Model file for the job. Use its own axes, mm. A direction names the side the tool comes from. Give positions to 0.01 mm unless a question says otherwise; leave off trailing zeros. Write each loop counter-clockwise with the first axis right and the second up, starting at its lowest first coordinate (ties: lowest second). Pieces come first, ordered by that corner, then holes. Notation, with made-up numbers: (86.5, -13.75) - (124.5, -13.75) arc R20 cw to (124.5, 11.25) - close; hole circle Ø8 at (61, 7.25). An arc over 180 degrees is marked (long way). Use CSV: the item, a comma, the result in double quotes.
from build123d import *

# Parameters (mm, degrees)
SKETCH1_W           = 38.1
SKETCH1_H           = 31.75
BOSS_EXTRUDE1_DEPTH = 14.732
SKETCH2_R           = 3.5687
BOSS_EXTRUDE2_DEPTH = 9.5758
SKETCH3_R           = 1.3462
CUT_EXTRUDE1_DEPTH  = 8.89


with BuildPart() as part:
    # Sketch1 → Boss-Extrude1 (new body)
    with BuildSketch(Plane.XY):
        with Locations((19.05, 15.875)):
            Rectangle(SKETCH1_W, SKETCH1_H)
    extrude(amount=BOSS_EXTRUDE1_DEPTH)

    # Sketch2 → Boss-Extrude2 (add)
    with BuildSketch(Plane(origin=(0, 0, 0), x_dir=(-1, 0, 0), z_dir=(0, 0, -1))):
        with Locations(Location((-35.56, 2.54, 0), (0, 0, 224.623028882))):
            Circle(SKETCH2_R)
        with Locations(Location((-2.54, 2.54, 0), (0, 0, 225.376971118))):
            Circle(SKETCH2_R)
        with Locations(Location((-35.56, 29.21, 0), (0, 0, 135.376971118))):
            Circle(SKETCH2_R)
        with Locations(Location((-2.54, 29.21, 0), (0, 0, 134.623028882))):
            Circle(SKETCH2_R)
    extrude(amount=BOSS_EXTRUDE2_DEPTH)

    # Sketch3 → Cut-Extrude1 (cut)
    with BuildSketch(Plane(origin=(0, 0, -9.5758), x_dir=(-1, 0, 0), z_dir=(0, 0, -1))):
        with Locations((-35.56, 29.21)):
            Circle(SKETCH3_R)
        with Locations((-2.54, 29.21)):
            Circle(SKETCH3_R)
        with Locations((-2.54, 2.54)):
            Circle(SKETCH3_R)
        with Locations((-35.56, 2.54)):
            Circle(SKETCH3_R)
    extrude(amount=-CUT_EXTRUDE1_DEPTH, mode=Mode.SUBTRACT)


solid = part.part
(1) Wall check: probe 1 along Y at (x, z) = (2.54, -6); probe 2 along X at (y, z) = (30, -4); probe 3 along Y at (x, z) = (28.5, 11.75). Give the ranges that are in metal, low to high. Write a range as [from, to].
Checked values:
probe 1,"y = [-1.03, 1.19], [3.89, 6.11], [25.64, 27.86], [30.56, 32.78]"
probe 2,"x = [-0.94, 1.45], [3.63, 6.02], [32.08, 34.47], [36.65, 39.04]"
probe 3,"y = [0, 31.75]"
(2) 3-axis set-ups, long thin cutter, end or side, ignore diameter. For faces 1 (the face through (35.6, -0.4, 0)), 2 (the face through (36, 3, -0.686)), 3 (the face through (38.5, 29.2, 0)), 4 (the face through (3, 32, 0)), 5 (the face through (-0.5, 29.3, 0)): which of +Z, -Z, +X, -X, +Y, -Y reach the whole face in a straight line?
Checked values:
face 1,"+Z, +X, -X, -Y"
face 2,"-Z"
face 3,"+Z, +X, +Y, -Y"
face 4,"+Z, +X, -X, +Y"
face 5,"+Z, -X, +Y, -Y"
(3) Saw through at B-B, the plane y = 2.54. List the corners of the cut face in (x, z), then the cut area to 3 significant figures.
Checked values:
outline,"(-1.03, -9.58) - (1.19, -9.58) - (1.19, -0.69) - (3.89, -0.69) - (3.89, -9.58) - (6.11, -9.58) - (6.11, 0) - (31.99, 0) - (31.99, -9.58) - (34.21, -9.58) - (34.21, -0.69) - (36.91, -0.69) - (36.91, -9.58) - (39.13, -9.58) - (39.13, 0) - (38.1, 0) - (38.1, 14.73) - (0, 14.73) - (0, 0) - (-1.03, 0) - close"
area,"650 mm^2"
(4) Flat gauge pins, fed straight in: P1, Ø1.1, axis at x = 34.5, y = 32.5, coming from the +Z side; P2, Ø2, axis at x = 6, z = -6, coming from the +Y side; P3, Ø2, axis at x = 10.5, z = 11.5, coming from the +Y side. Where does each tip first touch, or does it go through?
Checked values:
P1,"stops at z = 0"
P2,"stops at y = 31.8"
P3,"stops at y = 31.75"
(5) Saw through at C-C, the plane x = 2.54. List the corners of the cut face in (y, z).
Checked values:
outline,"(-1.03, -9.58) - (1.19, -9.58) - (1.19, -0.69) - (3.89, -0.69) - (3.89, -9.58) - (6.11, -9.58) - (6.11, 0) - (25.64, 0) - (25.64, -9.58) - (27.86, -9.58) - (27.86, -0.69) - (30.56, -0.69) - (30.56, -9.58) - (32.78, -9.58) - (32.78, 0) - (31.75, 0) - (31.75, 14.73) - (0, 14.73) - (0, 0) - (-1.03, 0) - close"
(6) Saw through at D-D, the plane z = 3.25. List the corners of the cut face in (x, y), then the cut area to 3 significant figures.
Checked values:
outline,"(0, 0) - (38.1, 0) - (38.1, 31.75) - (0, 31.75) - close"
area,"1,210 mm^2"
(7) Saw through at A-A, the plane z = -1.5. List the corners of the cut face in (x, y), then the cut area to 3 significant figures.
Checked values:
outline,"circle Ø7.14 at (2.54, 2.54); circle Ø7.14 at (2.54, 29.21); circle Ø7.14 at (35.56, 2.54); circle Ø7.14 at (35.56, 29.21); hole circle Ø2.69 at (2.54, 2.54); hole circle Ø2.69 at (2.54, 29.21); hole circle Ø2.69 at (35.56, 2.54); hole circle Ø2.69 at (35.56, 29.21)"
area,"137 mm^2"
(8) Pull direction Y, two halves, no side cores. Call faces 6 (the face through (38.956, 3.637, -4.721)), 7 (the face through (19, 16, 14.732)): released by +Y, released by -Y, zero draft, split by the parting line, or undercut.
Checked values:
face 6,"undercut"
face 7,"zero draft"
